Geometry: final body of the model. Coordinates: model frame, mm. A direction names the side the tool comes from. Give positions to 0.01 mm unless a question says otherwise; leave off trailing zeros. Order: outer loops, then holes, each group sorted by start corner. A loop starts at its lowest first (then second) coordinate and runs counter-clockwise, first axis right, second up. Notation, with made-up numbers: (45, 61.5) - (52, 61.5) arc R16 ccw to (52, 67.5) - close; hole circle Ø5 at (74, -39.75). An arc over 180 degrees is marked (long way). Write item = value, one per line. Start each with the question number.
from build123d import *

# Parameters (mm, degrees)
F1_DEPTH = 9
F2_DEPTH = 29
F4_DEPTH = 9
F5_DEPTH = 9
F0_W     = 50
F0_H     = 9
F6_DEPTH = 24
F7_R     = 5.5
F8_DEPTH = 9.001


with BuildPart() as f1:
    # F0 (on Front) → F1 (new body)
    with BuildSketch(Plane.XZ):
        Polygon((50, 9), (50, 0), (86.8198051534, 53.3933982822), (80.4558441227, 47.0294372515), (59.2426406871, 68.2426406871), (0, 9), align=None)
    extrude(amount=F1_DEPTH)

    # F0 (on Front) → F2 (join)
    with BuildSketch(Plane.XZ):
        Polygon((80.4558441227, 47.0294372515), (86.8198051534, 53.3933982822), (65.6066017178, 74.6066017178), (59.2426406871, 68.2426406871), align=None)
    extrude(amount=F2_DEPTH)

    # F3 (on face) → F4 (join)
    with BuildSketch(Plane(origin=(70.1066017178, 0, 70.1066017178), x_dir=(0.7071067812, 0, -0.7071067812), z_dir=(0.7071067812, 0, 0.7071067812))):
        with BuildLine():
            Line((23.6360389693, -29), (15.6360389693, -29))
            ThreePointArc((15.6360389693, -29), (8.6360389693, -36), (1.6360389693, -29))
            Line((1.6360389693, -29), (-6.3639610307, -29))
            ThreePointArc((-6.3639610307, -29), (8.6360389693, -44), (23.6360389693, -29))
        make_face()
    extrude(amount=-F4_DEPTH)

    # F3 (on face) → F5 (cut)
    with BuildSketch(Plane(origin=(70.1066017178, 0, 70.1066017178), x_dir=(0.7071067812, 0, -0.7071067812), z_dir=(0.7071067812, 0, 0.7071067812))):
        with BuildLine():
            Line((1.6360389693, -29), (15.6360389693, -29))
            ThreePointArc((15.6360389693, -29), (8.6360389693, -22), (1.6360389693, -29))
        make_face()
    extrude(amount=-F5_DEPTH, mode=Mode.SUBTRACT)

    # F0 (on Front) → F6 (join)
    with BuildSketch(Plane.XZ):
        with Locations((25, 4.5)):
            Rectangle(F0_W, F0_H)
    extrude(amount=F6_DEPTH)

    # F7 (on face) → F8 (cut, through all)
    with BuildSketch(Plane.XY.offset(9)):
        with Locations((8.5, -16.5)):
            Circle(F7_R)
        with Locations((41.5, -16.5)):
            Circle(F7_R)
    extrude(amount=-F8_DEPTH, mode=Mode.SUBTRACT)


solid = f1.part
Q1. Contact query for flat-ended pins moving along their axis: pin 1 (10 mm diameter, centred on x = 61.5, y = -35, fed in from -Z); pin 2 (1.5 mm diameter, centred on y = -25.5, z = 48.5, fed in from -X); pin 3 (4.5 mm diameter, centred on x = 17, z = 3.5, fed in from -Y). Output: stop coordinate, or through.
Q2. Pull-direction query (Y, two-part tool) for faces 1 (the cylindrical face through (72.003, -22.166, 61.936)), 2 (the flat face through (76.065, -16.803, 64.148)), 3 (the flat face through (43, 0, 30)); classes: +Y half, -Y half, draft (parallel to the pull), parting line (faces both ways), or undercut.
Q3. Section D-D, the plane z = 6.5. Return the cut outline in (x, y), then the cut area to 3 significant figures.
Q4. Material intervals for line 1 along X through (y, z) = (-16, 6); line 2 along Y through (x, z) = (41, 6); line 3 along Y through (x, z) = (68, 39), sorted ascending. Write a range as from..to.
Q5. Section B-B, the plane x = 8.5. Return the cut outline in (y, z), then the cut area to 4 significant figures.
Q6. Section C-C, the plane y = -27.5. Return the cut outline in (x, z).
Q7. Section A-A, the plane y = -16.5. Return the cut outline in (x, z).
Q8. Set-up query: faces 4 (the flat face through (25, -16, 9)), 5 (the flat face through (50, -16, 4)), 6 (the flat face through (83.593, -18.86, 50.167)). Return all of +Z, -Z, +X, -X, +Y, -Y with unobstructed straight access to the full face (end or side cutting, diameter ignored); none if empty.
The answers:
q1.pin_1 = 60.99
q1.pin_2 = 78.24
q1.pin_3 = -24
q2.face_1 = undercut
q2.face_2 = draft
q2.face_3 = +Y half
q3.outline = (0, -24) - (50, -24) - (50, -9) - (54.48, -9) - (54.48, 0) - (0, 0) - close; hole circle Ø11 at (8.5, -16.5); hole circle Ø11 at (41.5, -16.5)
q3.area = 1,050 mm²
q4.line_1 = 0..3.02, 13.98..36.02, 46.98..50
q4.line_2 = -24..-21.98, -11.02..0
q4.line_3 = -9..0
q5.outline = (-24, 0) - (-22, 0) - (-22, 9) - (-24, 9) - close; (-11, 0) - (0, 0) - (0, 17.5) - (-9, 17.5) - (-9, 9) - (-11, 9) - close
q5.area = 193.5 mm²
q6.outline = (59.24, 68.24) - (65.01, 62.47) - (71.38, 68.83) - (65.61, 74.61) - close; (74.68, 52.8) - (80.46, 47.03) - (86.82, 53.39) - (81.05, 59.17) - close
q7.outline = (0, 0) - (3, 0) - (3, 9) - (0, 9) - close; (14, 0) - (36, 0) - (36, 9) - (14, 9) - close; (47, 0) - (50, 0) - (50, 9) - (47, 9) - close; (59.24, 68.24) - (80.46, 47.03) - (86.82, 53.39) - (65.61, 74.61) - close
q8.face_4 = +Z, +X, -X, -Y
q8.face_5 = +Z, -Z, +X, -Y
q8.face_6 = -Z, +X, -Y
